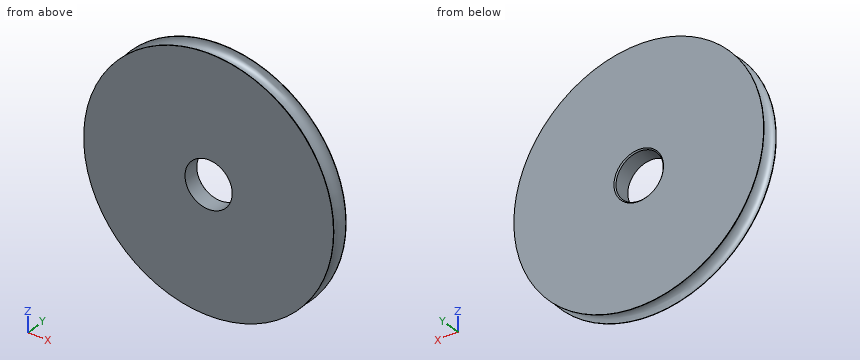
```python
from build123d import *

# Parameters (mm, degrees)
F0_R     = 21.425
F0_R_2   = 4.05
F1_DEPTH = 1.5
F4_SIZE  = 0.2


with BuildPart() as f1:
    # F0 (on Front) → F1 (new body, symmetric)
    with BuildSketch(Plane.XZ):
        Circle(F0_R)
        Circle(F0_R_2, mode=Mode.SUBTRACT)
    extrude(amount=F1_DEPTH, both=True)

    # F2 (on Right) → F3 (revolve, cut)
    with BuildSketch(Plane.YZ):
        with BuildLine():
            ThreePointArc((-1.425, 21.425), (-1.007627, 20.417373), (0, 20))
            Line((0, 20), (0, 21.425))
            Line((0, 21.425), (-1.425, 21.425))
        make_face()
        with BuildLine():
            Line((0, 21.425), (0, 20))
            ThreePointArc((0, 20), (1.007627, 20.417373), (1.425, 21.425))
            Line((1.425, 21.425), (0, 21.425))
        make_face()
    revolve(axis=Axis((0, -4.904328, 0), (0, -1, 0)), mode=Mode.SUBTRACT)

    # F4
    f4_edges = [f1.edges().sort_by_distance(p)[0] for p in [
        (-4.05, 1.5, 0),
    ]]
    chamfer(f4_edges, length=F4_SIZE)


solid = f1.part
```
Geometry: final body of the model. Coordinates: model frame, mm. Round coordinates to 2 decimals unless told otherwise and drop trailing zeros. Order: outer loops, then holes, each group sorted by start corner. A loop starts at its lowest first (then second) coordinate and runs counter-clockwise, first axis right, second up. Notation, with made-up numbers: (-12, 19) -> (23, 19) arc R25 ccw to (23, 31) -> close; hole circle Ø8 at (39, 83). An arc over 180 degrees is marked (long way). Use CSV: the item, a comma, the result in double quotes. Start each with the question number.
1) Section C-C (y = 0.7). Return the cut outline in (x, z), and give its area (3 significant figures).
2) Section B-B (x = 0). Return the cut outline in (y, z) (3 decimals), and give its area (3 significant figures).
3) Section A-A (z = 0). Return the cut outline in (x, y) (3 decimals).
4) Material intervals for line 1 along Z through (x, y) = (0, 0.55); line 2 along X through (y, z) = (-0.9, 1); line 3 along Z through (x, y) = (0, -0.1), sorted ascending. Write a range as from..to.
Returned:
1,outline,"circle Ø40.37 at (0, 0); hole circle Ø8.1 at (0, 0)"
1,area,"1,230 mm²"
2,outline,"(-1.5, -21.425) -> (-1.425, -21.425) arc R1.425 cw to (0, -20) arc R1.425 cw to (1.425, -21.425) -> (1.5, -21.425) -> (1.5, -4.25) -> (1.3, -4.05) -> (-1.5, -4.05) -> close; (-1.5, 4.05) -> (1.3, 4.05) -> (1.5, 4.25) -> (1.5, 21.425) -> (1.425, 21.425) arc R1.425 cw to (0, 20) arc R1.425 cw to (-1.425, 21.425) -> (-1.5, 21.425) -> close"
2,area,"97.8 mm²"
3,outline,"(-21.425, -1.5) -> (-4.05, -1.5) -> (-4.05, 1.3) -> (-4.25, 1.5) -> (-21.425, 1.5) -> (-21.425, 1.425) arc R1.425 cw to (-20, 0) arc R1.425 cw to (-21.425, -1.425) -> close; (4.05, -1.5) -> (21.425, -1.5) -> (21.425, -1.425) arc R1.425 cw to (20, 0) arc R1.425 cw to (21.425, 1.425) -> (21.425, 1.5) -> (4.25, 1.5) -> (4.05, 1.3) -> close"
4,line 1,"z = -20.11..-4.05, 4.05..20.11"
4,line 2,"x = -20.3..-3.92, 3.92..20.3"
4,line 3,"z = -20..-4.05, 4.05..20"
